Work out the finished part from the listing and answer in its coordinate system (mm). Round coordinates to 2 decimals unless told otherwise and drop trailing zeros. Write each loop counter-clockwise with the first axis right and the second up, starting at its lowest first coordinate (ties: lowest second). Pieces come first, ordered by that corner, then holes.
1. A flat-ended cylindrical pin translates along its axis: pin 1 Ø1.4 at (x, z) = (-6.96, 4.88) entering from -Y. Find the tip coordinate at first contact, or state that the pin passes through.
2. Find section D-D (y = 1.05). Write down the section's boundary in (x, z).
3. Find section A-A (z = -5). Write down the section's boundary in (x, y), and give its area (3 significant figures).
4. Straight lines are drawn through the part: probe 1 along X at (y, z) = (1.3, 0.5); probe 2 along X at (y, z) = (0.55, 0); probe 3 along X at (y, z) = (1, -1.5). For each, find the intervals that lie inside material, in ascending order.
5. Find section B-B (x = 70). Write down the section's boundary in (y, z), and give its area (3 significant figures).
6. Find section C-C (z = 0). Write down the section's boundary in (x, y), and give its area (3 significant figures).
```python
from build123d import *

# Parameters (mm, degrees)
ESQUISSE1_R             = 4
ESQUISSE1_R_2           = 1.2
BOSS_EXTRU_1_DEPTH      = 1.5
ESQUISSE2_R             = 1.2
ENL_V_MAT_EXTRU_1_DEPTH = 77.560702478


with BuildPart() as part:
    # Esquisse1 → Boss.-Extru.1 (new body)
    with BuildSketch(Plane(origin=(0, 0, 0), x_dir=(1, 0, 0), z_dir=(0, 1, 0))):
        with BuildLine():
            Line((7.702709274, -9.201536276), (15.560016707, -2.624096052))
            ThreePointArc((15.560016707, -2.624096052), (41.546598932, 6.702908226), (67.385064935, -3.026898513))
            ThreePointArc((67.385064935, -3.026898513), (73.026898513, -2.614935065), (72.614935065, 3.026898513))
            ThreePointArc((72.614935065, 3.026898513), (34.4702408, 19.282589401), (-6.02615989, 10.377157462))
            ThreePointArc((-6.02615989, 10.377157462), (-9.825172598, -6.889556112), (7.702709274, -9.201536276))
        make_face()
        with Locations(Location((0, 0, 0), (0, 0, 270))):
            Circle(ESQUISSE1_R, mode=Mode.SUBTRACT)
        with Locations(Location((70, 0, 0), (0, 0, 270))):
            Circle(ESQUISSE1_R_2, mode=Mode.SUBTRACT)
    extrude(amount=BOSS_EXTRU_1_DEPTH)

    # Esquisse2 → Enlèv. mat.-Extru.1 (cut, through all)
    with BuildSketch(Plane(origin=(0, 1.5, 0), x_dir=(1, 0, 0), z_dir=(0, 1, 0))):
        with Locations(Location((-6.959497257, -4.880102246, 0), (0, 0, 270))):
            Circle(ESQUISSE2_R)
        with Locations(Location((6.959497257, 4.880102246, 0), (0, 0, 270))):
            Circle(ESQUISSE2_R)
    extrude(amount=-ENL_V_MAT_EXTRU_1_DEPTH, mode=Mode.SUBTRACT)


solid = part.part
```
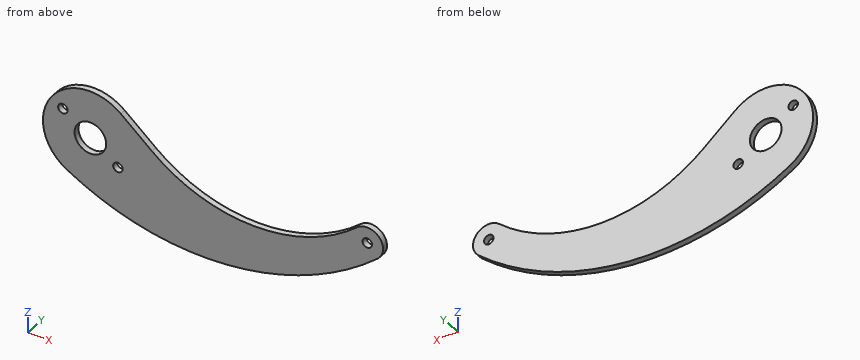
Worked answers:
1. pin 1: passes through
2. outline: (-6.03, -10.38) arc R68.03 ccw to (72.61, -3.03) arc R4 ccw to (67.39, 3.03) arc R40 cw to (15.56, 2.62) - (7.7, 9.2) arc R12 ccw (long way) to start; hole circle Ø2.4 at (-6.96, 4.88); hole circle Ø8 at (0, 0); hole circle Ø2.4 at (6.96, -4.88); hole circle Ø2.4 at (70, 0)
3. outline: (-10.91, 0) - (5.77, 0) - (5.77, 1.5) - (-10.91, 1.5) - close; (8.15, 0) - (29.68, 0) - (29.68, 1.5) - (8.15, 1.5) - close; (52.79, 0) - (70.22, 0) - (70.22, 1.5) - (52.79, 1.5) - close
3. area: 83.5 mm2
4. probe 1: x = -11.99 to -3.97, 3.97 to 18.34, 64.14 to 68.91, 71.09 to 73.97
4. probe 2: x = -12 to -4, 4 to 19.07, 63.4 to 68.8, 71.2 to 74
4. probe 3: x = -11.91 to -3.71, 3.71 to 21.51, 60.97 to 73.71
5. outline: (0, -5.17) - (1.5, -5.17) - (1.5, -1.2) - (0, -1.2) - close; (0, 1.2) - (1.5, 1.2) - (1.5, 4) - (0, 4) - close
5. area: 10.2 mm2
6. outline: (-12, 0) - (-4, 0) - (-4, 1.5) - (-12, 1.5) - close; (4, 0) - (19.07, 0) - (19.07, 1.5) - (4, 1.5) - close; (63.4, 0) - (68.8, 0) - (68.8, 1.5) - (63.4, 1.5) - close; (71.2, 0) - (74, 0) - (74, 1.5) - (71.2, 1.5) - close
6. area: 46.9 mm2
